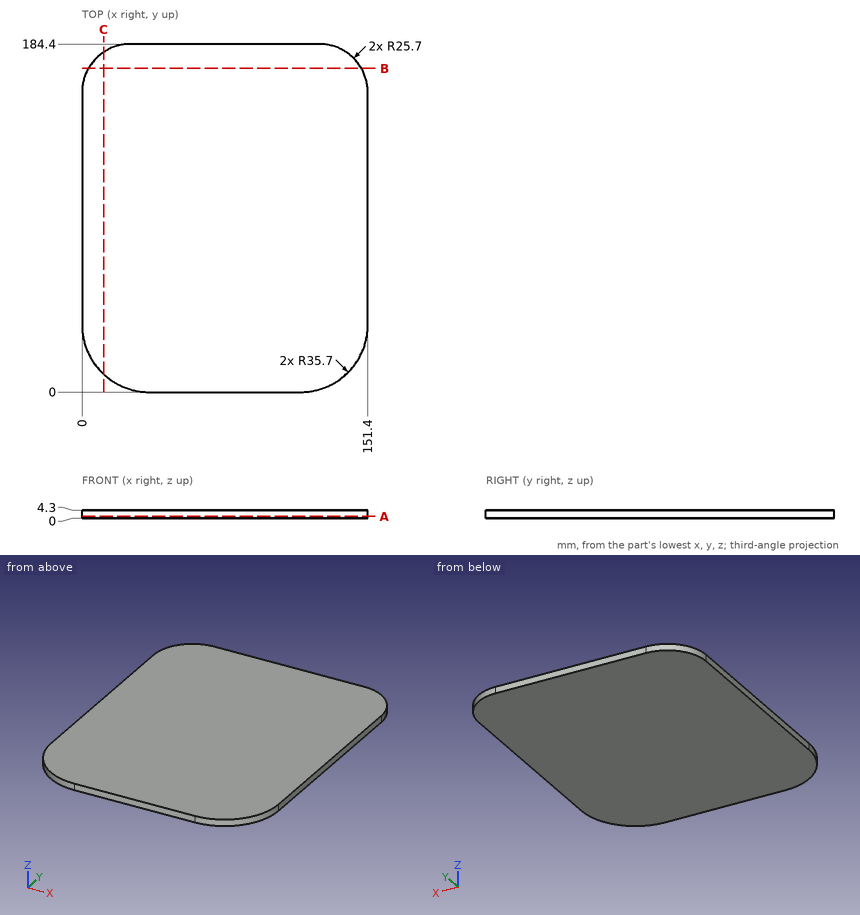
Input: dimensioned drawing with shaded views. Units: mm. Origin: part minimum x, y, z. Give positions to 0.01 mm unless a question says otherwise; leave off trailing zeros. Write each loop counter-clockwise with the first axis right and the second up, starting at its lowest first coordinate (ties: lowest second). Pieces come first, ordered by that corner, then holes. Notation, with made-up numbers: M 64.5,35 L 112.5,35 A25 ccw 112.5,69 Z; hole C -20,-23 d1. An arc over 180 degrees is marked long. Return JSON: item names as keys, results as strings. Group by question number.
1) Material intervals for line 1 along X through (y, z) = (35, 3.9); line 2 along Y through (x, z) = (131, 1.9); line 3 along Y through (x, z) = (140, 4), sorted ascending. Write a range as [from, to].
2) Cut plane B-B, the plane y = 171.5. Output: boundary loops of the cut face in (x, z).
3) Cut plane C-C, the plane x = 11.5. Output: boundary loops of the cut face in (y, z), plus the area to 3 significant figures.
4) Cut plane A-A, the plane z = 1.05. Output: boundary loops of the cut face in (x, y).
Recorded:
{
 "1": {"line 1": "x = [0.01, 151.39]", "line 2": "y = [3.44, 183.85]", "line 3": "y = [9.55, 180.05]"},
 "2": {"outline": "M 3.41,0 L 147.99,0 L 147.99,4.3 L 3.41,4.3 Z"},
 "3": {"outline": "M 9.45,0 L 180.12,0 L 180.12,4.3 L 9.45,4.3 Z", "area": "734 mm²"},
 "4": {"outline": "M 0,35.7 A35.7 ccw 35.7,0 L 115.7,0 A35.7 ccw 151.4,35.7 L 151.4,158.7 A25.7 ccw 125.7,184.4 L 25.7,184.4 A25.7 ccw 0,158.7 Z"}
}
